CAD build for the part. Positions are in the model's coordinates, mm. A direction names the side the tool comes from. Round coordinates to 2 decimals unless told otherwise and drop trailing zeros. Order: outer loops, then holes, each group sorted by start corner. A loop starts at its lowest first (then second) coordinate and runs counter-clockwise, first axis right, second up. Notation, with made-up numbers: M 29,20.25 L 88,20.25 A20 cw 88,48.25 Z; hole C -5.75,-28.5 d2. An arc over 180 degrees is marked long. Answer as a JSON object with one key per item and string values.
Autodesk Inventor part; units mm, degrees
ref_plane "YZ Plane" through (0, 0, 0) normal (1, 0, 0) x (0, 1, 0)
ref_plane "XZ Plane" through (0, 0, 0) normal (0, 1, 0) x (-1, 0, 0)
ref_plane "XY Plane" through (0, 0, 0) normal (0, 0, 1) x (1, 0, 0)
sketch "Sketch1" plane through (0, 0, 0) normal (0, 0, 1) x (1, 0, 0)
  line L0 (0, 0) -> (12.5476, 0)
  line L1 (12.5476, 0) -> (12.5476, 12.5476)
  line L2 (12.5476, 12.5476) -> (0, 12.5476)
  line L3 (0, 12.5476) -> (0, 0)
  line L4 (1.5113, 1.5113) -> (11.0363, 1.5113)
  line L5 (11.0363, 1.5113) -> (11.0363, 11.0363)
  line L6 (11.0363, 11.0363) -> (1.5113, 11.0363)
  line L7 (1.5113, 11.0363) -> (1.5113, 1.5113)
  line L8 (1.5113, 1.5113) -> (11.0363, 11.0363) construction
  line L9 (11.0363, 1.5113) -> (1.5113, 11.0363) construction
  point P0 (6.2738, 6.2738)
  dimension "d0" = 12.5476
  dimension "d1" = 12.5476
  dimension "d2" = 9.525
  dimension "d3" = 9.525
extrude "Extrusion1" add sketch "Sketch1" along normal blind 381
sketch "Sketch2" plane through (12.5476, 0, 0) normal (1, 0, 0) x (0, 0, -1)
  circle A0 centre (-19.05, 6.2738) radius 2.413
  line L0 (0, 0) -> (0, 12.5476)
  dimension "d6" = 4.826
  dimension "d13" = 19.05
extrude "Extrusion2" cut sketch "Sketch2" against normal blind 419.1
sketch "Sketch3" plane through (12.5476, 0, 0) normal (1, 0, 0) x (0, 0, -1)
  circle A0 centre (-372.11, 6.2738) radius 2.413
  line L0 (-381, 0) -> (-381, 12.5476)
  dimension "d9" = 4.826
  dimension "d12" = 8.89
extrude "Extrusion3" cut sketch "Sketch3" against normal blind 25.4
sketch "Sketch5" plane through (0, 0, 0) normal (-1, 0, 0) x (0, 0, 1)
  circle A0 centre (19.05, 6.2738) radius 2.413
  circle A1 centre (11.05, 6.2738) radius 1.3462
  circle A2 centre (27.05, 6.2738) radius 1.3462
  line L0 (0, 12.5476) -> (381, 12.5476)
  line L1 (11.05, 6.2738) -> (27.05, 6.2738)
  line L2 (0, 12.5476) -> (0, 0)
  dimension "d14" = 2.6924
  dimension "d15" = 2.6924
  dimension "d16" = 16
  dimension "d19" = 11.05
  dimension "d20" = 19.05
  dimension "d21" = 27.05
extrude "Extrusion4" cut sketch "Sketch5" against normal blind 12.7 contours A1 | A2
properties part number "custom Box Aluminum" material "Aluminum 6061"
Item 1: Drop a flat-ended pin along its axis: pin 1 Ø1.6 at (y, z) = (6.27, 27.05) entering from +X. Give the stop position or say it passes through.
Worked answers:
{"pin 1": "passes through"}
Item 2: 3-axis set-ups, long thin cutter, end or side, ignore diameter. For faces 1 (the flat face through (0, 6, 188)), 2 (the flat face through (6, 1.511, 188)): which of +Z, -Z, +X, -X, +Y, -Y reach the whole face in a straight line?
Worked answers:
{"face 1": "+Z, -Z, -X, +Y, -Y", "face 2": "+Z, -Z"}
Item 3: Wall check: line 1 along X through (y, z) = (9.75, 169); line 2 along Y through (x, z) = (11.75, 19.05). Give the ranges that are in metal, low to high. Write a range as [from, to].
Worked answers:
{"line 1": "x = [0, 1.51], [11.04, 12.55]", "line 2": "y = [0, 3.86], [8.69, 12.55]"}
Item 4: Two-plate mould, pull along X, no slides. Class faces 3 (the flat face through (6, 11.036, 188)), 4 (the flat face through (1, 6, 381)), 5 (the flat face through (12.548, 6, 188)): released by +X, released by -X, zero draft, split by the parting line, or undercut.
Worked answers:
{"face 3": "undercut", "face 4": "zero draft", "face 5": "released by +X"}
Item 5: Saw through at B-B on z = 267. List the corners of the cut face in (x, y), and give its area (3 significant figures).
Worked answers:
{"outline": "M 0,0 L 12.55,0 L 12.55,12.55 L 0,12.55 Z; hole M 1.51,1.51 L 11.04,1.51 L 11.04,11.04 L 1.51,11.04 Z", "area": "66.7 mm2"}
Item 6: Saw through at A-A on x = 5.25. List the corners of the cut face in (y, z), and give its area (3 significant figures).
Worked answers:
{"outline": "M 0,0 L 1.51,0 L 1.51,381 L 0,381 Z; M 11.04,0 L 12.55,0 L 12.55,381 L 11.04,381 Z", "area": "1,150 mm2"}
